The model under review builds one solid part; all positions refer to its coordinate system, in mm. Face numbers are marked on the shaded views. A direction names the side the tool comes from. Give positions to 0.01 mm unless a question says otherwise; leave off trailing zeros. Loops run counter-clockwise (first coordinate to the right, second up) from the corner with the lowest first, then second, coordinate; pieces in that order, holes last. Notation, with made-up numbers: M 81,23 L 91,23 A4 ccw 91,27 Z; hole C 6,-35 d8. An arc over 180 degrees is marked long. Return JSON: item names as keys, results as strings.
Autodesk Inventor part; units mm, degrees
ref_plane "YZ Plane" through (0, 0, 0) normal (1, 0, 0) x (0, 1, 0)
ref_plane "XZ Plane" through (0, 0, 0) normal (0, 1, 0) x (-1, 0, 0)
ref_plane "XY Plane" through (0, 0, 0) normal (0, 0, 1) x (1, 0, 0)
sketch "Sketch10" plane through (0, 0, 0) normal (0, 1, 0) x (-1, 0, 0)
  circle A0 centre (0, 0) radius 1.6
  arc A1 (0.7577, 7.4616) -> (-3.1789, -6.793) centre (0, 0) ccw
  line L0 (0, 0) -> (0, -7.5) construction
  line L1 (0, 0) -> (7.5, 0) construction
  line L2 (0, 0) -> (63.5588, 0) construction
  line L3 (40, 0) -> (20, 0)
  line L4 (20, 0) -> (20, -10.3)
  line L5 (20, -10.3) -> (40, -10.3)
  line L6 (40, -10.3) -> (40, -15.3)
  line L7 (40, -15.3) -> (19.4481, -15.3)
  line L8 (10.9712, -13.4147) -> (-3.1789, -6.793)
  line L9 (40, 0) -> (40, 5)
  line L10 (40, 5) -> (29.0513, 5)
  line L11 (20.9694, 5.4093) -> (0.7577, 7.4616)
  arc A2 (20.9694, 5.4093) -> (29.0513, 5) centre (29.0513, 85) ccw
  arc A3 (10.9712, -13.4147) -> (19.4481, -15.3) centre (19.4481, 4.7) ccw
  point P0 (15, -15.3)
  point P1 (25, 5)
  dimension "d117" = 3.2
  dimension "d118" = 15
  dimension "d120" = 10.3
  dimension "d121" = 20
  dimension "d122" = 0
  dimension "d123" = 20
  dimension "d124" = 5
  dimension "d125" = 5
  dimension "d126" = 25
  dimension "d127" = 15
  dimension "d128" = 80
  dimension "d129" = 20
  dimension "d133" = 0
extrude "Extrusion7" add sketch "Sketch10" along normal blind 7
fillet "Fillet5" radius 2 4 edges at (-40, 3.5, 5) (-40, 3.5, 0) (-40, 3.5, -10.3) (-40, 3.5, -15.3)
properties part number "Soportes filamento"
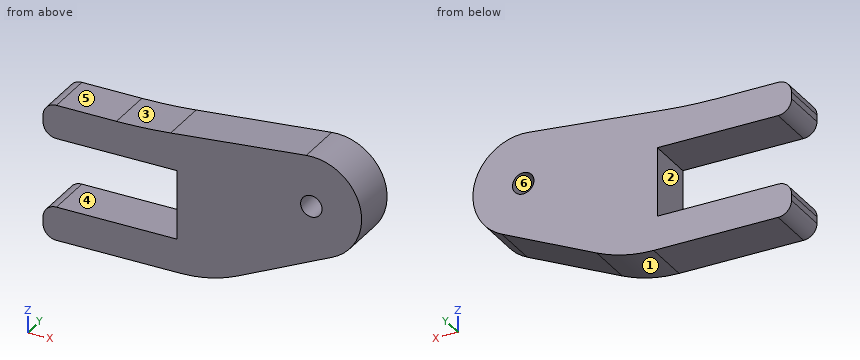
1) Consider section D-D on x = 0. Write out the cut boundary in (y, z).
From the geometry:
{"outline": "M 0,-8.28 L 7,-8.28 L 7,-1.6 L 0,-1.6 Z; M 0,1.6 L 7,1.6 L 7,7.5 L 0,7.5 Z"}
2) Consider section C-C on z = -8. Write out the cut boundary in (x, y).
From the geometry:
{"outline": "M -20,0 L 0.6,0 L 0.6,7 L -20,7 Z"}
3) Consider section A-A on x = -30. Write out the cut boundary in (y, z), then the cut area to 3 significant figures.
From the geometry:
{"outline": "M 0,-15.3 L 7,-15.3 L 7,-10.3 L 0,-10.3 Z; M 0,0 L 7,0 L 7,5 L 0,5 Z", "area": "70.0 mm²"}
4) Insertion check: pin 1 (1 mm diameter, centred on x = -1.5, y = 4.5, fed in from -Z); pin 2 (3.5 mm diameter, centred on x = -32, y = 4.5, fed in from +Z); pin 3 (4 mm diameter, centred on y = 1.5, z = -0.5, fed in from -X). Each pin has a flat end and moves straight along its axis. Give the tip position at first contact, or say it passes through.
From the geometry:
{"pin 1": "z = -9.22", "pin 2": "z = 5", "pin 3": "x = -39.94"}
5) Consider section B-B on y = 0.5. Write out the cut boundary in (x, z).
From the geometry:
{"outline": "M -40,-13.3 A2 ccw -38,-15.3 L -19.45,-15.3 A20 ccw -10.97,-13.41 L 3.18,-6.79 A7.5 ccw -0.76,7.46 L -20.97,5.41 A80.01 cw -29.05,5 L -38,5 A2 ccw -40,3 L -40,2 A2 ccw -38,0 L -20,0 L -20,-10.3 L -38,-10.3 A2 ccw -40,-12.3 Z; hole C 0,0 d3.2"}
6) The part is to be moulded in two halves that separate along Z. For the marked faces 1, 2 and 3, say which applies: released by +Z, released by -Z, zero draft, split by the parting line, or undercut.
From the geometry:
{"face 1": "released by -Z", "face 2": "undercut", "face 3": "released by +Z"}
7) Wall thickness on L1, parallel to Z at x = -23, y = 2; L2, parallel to Z at x = 0, y = 2.25; L3, parallel to X at y = 2.5, z = -1.25: over which ranges is each line inside the solid? List them lowest first. Write a range as from..to.
From the geometry:
{"L1": "-15.3..-10.3, 0..5.23", "L2": "-8.28..-1.6, 1.6..7.5", "L3": "-20..-1, 1..7.4"}
8) Tool access review of the marked faces 4, 5 and 6: name each direction out of +Z, -Z, +X, -X, +Y, -Y from which nothing blocks a thin tool from reaching the whole face with its end or side.
From the geometry:
{"face 4": "-X, +Y, -Y", "face 5": "+Z, -X, +Y, -Y", "face 6": "+Y, -Y"}
